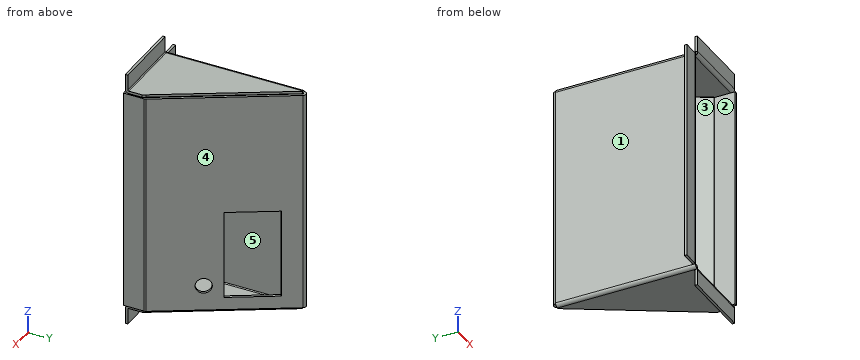
from build123d import *

# Parameters (mm, degrees)
CROQUIS3_W                         = 120
CROQUIS3_H                         = 175
BRIDA_BASE1_DEPTH                  = 2
BRIDA_START                        = -87.5
BRIDA_DE_ARISTA1_DEPTH             = 175
BRIDA_DE_ARISTA1_2_DEPTH           = 175
BRIDA_DE_ARISTA2_DEPTH             = 175
BRIDA_DE_ARISTA2_2_DEPTH           = 175
BRIDA_DE_ARISTA3_STRIP_CUT_DEPTH   = 109.78686976
BRIDA_DE_ARISTA3_STRIP_CUT_2_DEPTH = 109.78686976
BRIDA_DE_ARISTA3_DEPTH             = 109.78686976
BRIDA_DE_ARISTA3_BEND_DEPTH        = 109.78686976
CORTAR_EXTRUIR5_DEPTH              = 2
CORTAR_EXTRUIR6_DEPTH              = 2
BRIDA_DE_ARISTA4_STRIP_W           = 9.4732
BRIDA_DE_ARISTA4_STRIP_H           = 2
BRIDA_DE_ARISTA4_STRIP_CUT_DEPTH   = 56.268172105
BRIDA_DE_ARISTA4_STRIP_2_W         = 9.4732
BRIDA_DE_ARISTA4_STRIP_2_H         = 2
BRIDA_DE_ARISTA4_STRIP_CUT_2_DEPTH = 173.529368978
BRIDA_DE_ARISTA4_STRIP_3_W         = 9.4732
BRIDA_DE_ARISTA4_STRIP_3_H         = 2
BRIDA_DE_ARISTA4_STRIP_CUT_3_DEPTH = 56.268172105
BRIDA_DE_ARISTA4_DEPTH             = 56.268172105
BRIDA_DE_ARISTA4_BEND_DEPTH        = 173.529368978
BRIDA_DE_ARISTA4_BEND_2_DEPTH      = 56.268172105
CROQUIS37_R                        = 6
CROQUIS37_W                        = 70
CROQUIS37_H                        = 40
CORTAR_EXTRUIR7_DEPTH              = 2


# Read off the part's stored shape, not the designer's step: Brida de arista1, Brida de arista2
# Sheet-metal steps are written as plain solids
with BuildPart() as part:
    # Croquis3 → Brida base1 (new body)
    with BuildSketch(Plane(origin=(45, 25.980762114, 0), x_dir=(0.5000000000000044, -0.8660254037844362, 0), z_dir=(-0.8660254037844362, -0.5000000000000044, 0))):
        with Locations((-30, 0)):
            Rectangle(CROQUIS3_W, CROQUIS3_H)
    extrude(amount=-BRIDA_BASE1_DEPTH)

    # Brida de arista1 outline → Brida de arista1 (cut)
    with BuildSketch(Plane.XY.offset(BRIDA_START)):
        with BuildLine():
            Line((0, 103.923048454), (2.056713114, 100.360716845))
            ThreePointArc((2.056713114, 100.360716845), (3.797397716, 100.232553298), (5.10656512, 99.078218214))
            Line((5.10656512, 99.078218214), (1.732050808, 104.923048454))
            Line((1.732050808, 104.923048454), (0, 103.923048454))
        make_face()
    extrude(amount=BRIDA_DE_ARISTA1_DEPTH, mode=Mode.SUBTRACT)

    # Brida de arista1 2 outline → Brida de arista1 2 (add)
    with BuildSketch(Plane.XY.offset(BRIDA_START)):
        with BuildLine():
            ThreePointArc((2.056713114, 100.360716845), (0.574476274, 99.387476127), (0, 97.709918214))
            Line((0, 97.709918214), (0, -12.076951546))
            Line((0, -12.076951546), (2, -12.076951546))
            Line((2, -12.076951546), (2, 97.709918214))
            ThreePointArc((2, 97.709918214), (2.545953891, 98.421419178), (3.374514312, 98.078218214))
            Line((3.374514312, 98.078218214), (2.056713114, 100.360716845))
        make_face()
    extrude(amount=BRIDA_DE_ARISTA1_2_DEPTH)

    # Brida de arista2 outline → Brida de arista2 (cut)
    with BuildSketch(Plane.XY.offset(BRIDA_START)):
        with BuildLine():
            ThreePointArc((59.63336512, 4.63503024), (59.906752616, 3.975014439), (60, 3.26673024))
            Line((60, 3.26673024), (60, 0))
            Line((60, 0), (61.732050808, 1))
            Line((61.732050808, 1), (59.63336512, 4.63503024))
        make_face()
    extrude(amount=BRIDA_DE_ARISTA2_DEPTH, mode=Mode.SUBTRACT)

    # Brida de arista2 2 outline → Brida de arista2 2 (add)
    with BuildSketch(Plane.XY.offset(BRIDA_START)):
        with BuildLine():
            Line((60, -13), (60, 0))
            Line((60, 0), (57.901314312, 3.63503024))
            ThreePointArc((57.901314312, 3.63503024), (57.974900964, 3.457376349), (58, 3.26673024))
            Line((58, 3.26673024), (58, -13))
            Line((58, -13), (60, -13))
        make_face()
    extrude(amount=BRIDA_DE_ARISTA2_2_DEPTH)

    # Brida de arista3 strip (across the edge) → Brida de arista3 strip cut (cut)
    with BuildSketch(Plane(origin=(2, -12.076951546, -87.5), x_dir=(0.0017453283659016917, 0, 0.9999984769132877), z_dir=(0, 1, 0))):
        Polygon((-8.741361837, -1.984746476), (0.731823734, -2.001280321), (0.735314391, -0.001283367), (-8.73787118, 0.015250478), align=None)
    extrude(amount=BRIDA_DE_ARISTA3_STRIP_CUT_DEPTH, mode=Mode.SUBTRACT)

    # Brida de arista3 strip 2 (across the edge) → Brida de arista3 strip cut 2 (cut)
    with BuildSketch(Plane(origin=(2, 97.709918214, 87.5), x_dir=(0.0017453283659016917, 0, -0.9999984769132877), z_dir=(0, -1, 0))):
        Polygon((-8.741361837, -1.984746476), (0.731823734, -2.001280321), (0.735314391, -0.001283367), (-8.73787118, 0.015250478), align=None)
    extrude(amount=BRIDA_DE_ARISTA3_STRIP_CUT_2_DEPTH, mode=Mode.SUBTRACT)

    # Brida de arista3 section (across the edge) → Brida de arista3 (add)
    with BuildSketch(Plane(origin=(2, -12.076951546, -87.5), x_dir=(0.0017453283659016917, 0, 0.9999984769132877), z_dir=(0, 1, 0))):
        with BuildLine():
            Line((-2, 0.735315511), (-2, 57.003487616))
            Line((-2, 57.003487616), (0, 57.003487616))
            Line((0, 57.003487616), (0, 0.735315511))
            ThreePointArc((0, 0.735315511), (0.215290812, 0.214915386), (0.735314391, -0.001283367))
            Line((0.735314391, -0.001283367), (0.731823734, -2.001280321))
            ThreePointArc((0.731823734, -2.001280321), (-1.200156346, -1.198063504), (-2, 0.735315511))
        make_face()
    extrude(amount=BRIDA_DE_ARISTA3_DEPTH)

    # Brida de arista3 section 2 (across the edge) → Brida de arista3 bend (add)
    with BuildSketch(Plane(origin=(2, 97.709918214, 87.5), x_dir=(0.0017453283659016917, 0, -0.9999984769132877), z_dir=(0, -1, 0))):
        with BuildLine():
            Line((-2, 0.735315511), (-2, 57.003487616))
            Line((-2, 57.003487616), (0, 57.003487616))
            Line((0, 57.003487616), (0, 0.735315511))
            ThreePointArc((0, 0.735315511), (0.215290812, 0.214915386), (0.735314391, -0.001283367))
            Line((0.735314391, -0.001283367), (0.731823734, -2.001280321))
            ThreePointArc((0.731823734, -2.001280321), (-1.200156346, -1.198063504), (-2, 0.735315511))
        make_face()
    extrude(amount=BRIDA_DE_ARISTA3_BEND_DEPTH)

    # Croquis23 → Cortar-Extruir5 (cut)
    with BuildSketch(Plane(origin=(-0.156200564, 0, 89.496239762), x_dir=(0.9999984769132877, 0, 0.0017453283659016985), z_dir=(-0.0017453283659016987, 0, 0.9999984769132878))):
        Polygon((3.221792941, 98.078218214), (57.748509892, 3.63503024), (59.156200802, 1.196834349), (59.156200802, 97.709918214), align=None)
    extrude(amount=-CORTAR_EXTRUIR5_DEPTH, mode=Mode.SUBTRACT)

    # Croquis24 → Cortar-Extruir6 (cut)
    with BuildSketch(Plane(origin=(-0.156200564, 0, -89.496239762), x_dir=(-0.9999984769132877, 0, 0.001745328365901773), z_dir=(-0.0017453283659017733, 0, -0.9999984769132878))):
        Polygon((-3.527225405, 98.078218214), (-58.053942356, 3.63503024), (-59.156200802, 1.725859701), (-59.156200802, 97.709918214), align=None)
    extrude(amount=-CORTAR_EXTRUIR6_DEPTH, mode=Mode.SUBTRACT)

    # Brida de arista4 strip (across the edge) → Brida de arista4 strip cut (cut)
    with BuildSketch(Plane(origin=(58.999910138, -12.076951546, -89.599486758), x_dir=(0, 1, 0), z_dir=(-0.9999984769132877, -4.100332633432973e-15, 0.00174532836590182))):
        with Locations((-2, -1)):
            Rectangle(BRIDA_DE_ARISTA4_STRIP_W, BRIDA_DE_ARISTA4_STRIP_H)
    extrude(amount=BRIDA_DE_ARISTA4_STRIP_CUT_DEPTH, mode=Mode.SUBTRACT)

    # Brida de arista4 strip 2 (across the edge) → Brida de arista4 strip cut 2 (cut)
    with BuildSketch(Plane(origin=(0, -12.076951546, -86.764684489), x_dir=(0, 1, 0), z_dir=(0, 0, 1))):
        with Locations((-2, -1)):
            Rectangle(BRIDA_DE_ARISTA4_STRIP_2_W, BRIDA_DE_ARISTA4_STRIP_2_H)
    extrude(amount=BRIDA_DE_ARISTA4_STRIP_CUT_2_DEPTH, mode=Mode.SUBTRACT)

    # Brida de arista4 strip 3 (across the edge) → Brida de arista4 strip cut 3 (cut)
    with BuildSketch(Plane(origin=(2.731823734, -12.076951546, 89.501280321), x_dir=(0, 1, 0), z_dir=(0.9999984769132877, 2.0039219637078435e-15, 0.0017453283659018195))):
        with Locations((-2, -1)):
            Rectangle(BRIDA_DE_ARISTA4_STRIP_3_W, BRIDA_DE_ARISTA4_STRIP_3_H)
    extrude(amount=BRIDA_DE_ARISTA4_STRIP_CUT_3_DEPTH, mode=Mode.SUBTRACT)

    # Brida de arista4 section (across the edge) → Brida de arista4 (add)
    with BuildSketch(Plane(origin=(58.999910138, -12.076951546, -89.599486758), x_dir=(0, 1, 0), z_dir=(-0.9999984769132877, -4.100332633432973e-15, 0.00174532836590182))):
        with BuildLine():
            Line((0, 0.7366), (0, 13))
            Line((0, 13), (2, 13))
            Line((2, 13), (2, 0.7366))
            ThreePointArc((2, 0.7366), (2.215745145, 0.215745145), (2.7366, 0))
            Line((2.7366, 0), (2.7366, -2))
            ThreePointArc((2.7366, -2), (0.801531583, -1.198468417), (0, 0.7366))
        make_face()
    extrude(amount=BRIDA_DE_ARISTA4_DEPTH)

    # Brida de arista4 section 2 (across the edge) → Brida de arista4 bend (add)
    with BuildSketch(Plane(origin=(0, -12.076951546, -86.764684489), x_dir=(0, 1, 0), z_dir=(0, 0, 1))):
        with BuildLine():
            Line((0, 0.7366), (0, 13))
            Line((0, 13), (2, 13))
            Line((2, 13), (2, 0.7366))
            ThreePointArc((2, 0.7366), (2.215745145, 0.215745145), (2.7366, 0))
            Line((2.7366, 0), (2.7366, -2))
            ThreePointArc((2.7366, -2), (0.801531583, -1.198468417), (0, 0.7366))
        make_face()
    extrude(amount=BRIDA_DE_ARISTA4_BEND_DEPTH)

    # Brida de arista4 section 3 (across the edge) → Brida de arista4 bend 2 (add)
    with BuildSketch(Plane(origin=(2.731823734, -12.076951546, 89.501280321), x_dir=(0, 1, 0), z_dir=(0.9999984769132877, 2.0039219637078435e-15, 0.0017453283659018195))):
        with BuildLine():
            Line((0, 0.7366), (0, 13))
            Line((0, 13), (2, 13))
            Line((2, 13), (2, 0.7366))
            ThreePointArc((2, 0.7366), (2.215745145, 0.215745145), (2.7366, 0))
            Line((2.7366, 0), (2.7366, -2))
            ThreePointArc((2.7366, -2), (0.801531583, -1.198468417), (0, 0.7366))
        make_face()
    extrude(amount=BRIDA_DE_ARISTA4_BEND_2_DEPTH)

    # Croquis37 → Cortar-Extruir7 (cut)
    with BuildSketch(Plane(origin=(46.732050808, 26.980762114, 0), x_dir=(0, 0, -1), z_dir=(0.866025403784436, 0.5000000000000047, 0))):
        with Locations(Location((67.5, 14.250971375, 0), (0, 0, 90))):
            Circle(CROQUIS37_R)
        with Locations((42.5, 48.250971375)):
            Rectangle(CROQUIS37_W, CROQUIS37_H)
    extrude(amount=-CORTAR_EXTRUIR7_DEPTH, mode=Mode.SUBTRACT)


solid = part.part
The listing builds one solid part. Answer for the finished solid, in the listing's coordinates (mm). Face numbers are marked on the shaded views. A direction names the side the tool comes from. Coordinates: 2 decimals unless noted, no trailing zeros. Write each loop counter-clockwise with the first axis right and the second up, starting at its lowest first coordinate (ties: lowest second). Pieces come first, ordered by that corner, then holes. Notation, with made-up numbers: (85, 61) - (104, 61) arc R14 ccw to (104, 73) - close; hole circle Ø4 at (-32.75, -14.75). An arc over 180 degrees is marked (long way). Answer as CSV lines item,"result".
1. Given P1, Ø10, axis at y = 13.5, z = 31.5, coming from the +X side; P2, Ø4, axis at y = 75, z = 6.5, coming from the +X side; P3, Ø1.5, axis at x = 37, y = 8.5, coming from the +Z side, each flat-ended and moving along its own axis, determine where each tip first touches the part or whether it passes through.
Computed values:
P1,"stops at x = 57.4"
P2,"stops at x = 20.16"
P3,"stops at z = 89.56"
2. A tool of negligible diameter and unlimited length cuts with its end or side. For the marked faces 3, 4 and 5, from which of +Z, -Z, +X, -X, +Y, -Y can it reach the whole face along a straight path? Write none if from no direction.
Computed values:
face 3,"+Z, -Y"
face 4,"+Z, -Z, +X, +Y"
face 5,"-Y"
3. Straight lines are drawn through the part: line 1 (Z direction, x = 40, y = 13); line 2 (Z direction, x = 11.5, y = -5.5); line 3 (X direction, y = -7, z = -70). For each, find the intervals that lie inside material, in ascending order. Write a range as [from, to].
Computed values:
line 1,"z = [-89.57, -87.57], [87.57, 89.57]"
line 2,"z = [-89.52, -87.52], [87.52, 89.52]"
line 3,"x = [0, 2], [58, 60]"
4. Find section A-A (z = -11). Give the vertices of the cut face in (x, y), plus the area to 3 significant figures.
Computed values:
outline,"(-13, -12.08) - (-0.74, -12.08) arc R2.74 ccw to (2, -9.34) - (2, 97.71) arc R0.74 cw to (3.37, 98.08) - (10.87, 85.09) - (12.61, 86.09) - (5.11, 99.08) arc R2.74 ccw to (0, 97.71) - (0, -9.34) arc R0.74 cw to (-0.74, -10.08) - (-13, -10.08) - close; (30.87, 50.45) - (57.9, 3.64) arc R0.74 cw to (58, 3.27) - (58, -13) - (60, -13) - (60, 3.27) arc R2.74 ccw to (59.63, 4.64) - (32.61, 51.45) - close"
area,"426 mm²"
5. Find section B-B (y = 81). Give the vertices of the cut face in (x, z).
Computed values:
outline,"(0, -86.76) arc R2.74 ccw to (2.73, -89.5) - (13.23, -89.52) - (13.23, -87.52) - (2.74, -87.5) arc R0.74 cw to (2, -86.76) - (2, 86.76) arc R0.74 cw to (2.74, 87.5) - (12.93, 87.52) - (12.93, 89.52) - (2.73, 89.5) arc R2.74 ccw to (0, 86.76) - close; (13.23, -87.5) - (15.54, -87.5) - (15.54, -77.5) - (13.23, -77.5) - close; (13.23, -7.5) - (15.54, -7.5) - (15.54, 87.5) - (13.23, 87.5) - close"
6. Determine the mould class of the marked faces 1 and 2 for opening direction Z: +Z half, -Z half, draft (parallel to the pull), parting line (faces both ways), or undercut.
Computed values:
face 1,"draft"
face 2,"undercut"
7. Find section D-D (z = 28.5). Give the vertices of the cut face in (x, y).
Computed values:
outline,"(-13, -12.08) - (-0.74, -12.08) arc R2.74 ccw to (2, -9.34) - (2, 97.71) arc R0.74 cw to (3.37, 98.08) - (57.9, 3.64) arc R0.74 cw to (58, 3.27) - (58, -13) - (60, -13) - (60, 3.27) arc R2.74 ccw to (59.63, 4.64) - (5.11, 99.08) arc R2.74 ccw to (0, 97.71) - (0, -9.34) arc R0.74 cw to (-0.74, -10.08) - (-13, -10.08) - close"
8. Find section C-C (y = 48). Give the vertices of the cut face in (x, z).
Computed values:
outline,"(0, -86.76) arc R2.74 ccw to (2.73, -89.5) - (32.28, -89.55) - (32.29, -87.55) - (2.74, -87.5) arc R0.74 cw to (2, -86.76) - (2, 86.76) arc R0.74 cw to (2.74, 87.5) - (31.98, 87.55) - (31.98, 89.55) - (2.73, 89.5) arc R2.74 ccw to (0, 86.76) - close; (32.29, -87.5) - (34.6, -87.5) - (34.6, 87.5) - (32.29, 87.5) - close"
